The model under review builds one solid part; all positions refer to its coordinate system, in mm. Face numbers are marked on the shaded views. A direction names the side the tool comes from. Coordinates: 2 decimals unless noted, no trailing zeros. Order: outer loops, then holes, each group sorted by start corner. A loop starts at its lowest first (then second) coordinate and runs counter-clockwise, first axis right, second up. Notation, with made-up numbers: M 73,-10.5 L 80,-10.5 A32 ccw 80,23.5 Z; hole C 52.5,76.5 d11. An arc over 180 degrees is marked long. One line per item, written item: value.
```python
from build123d import *

# Parameters (mm, degrees)
SKETCH1_R           = 1.5
BOSS_EXTRUDE1_DEPTH = 2
SKETCH2_R           = 4
SKETCH2_R_2         = 3
BOSS_EXTRUDE2_DEPTH = 3


with BuildPart() as part:
    # Sketch1 → Boss-Extrude1 (new body)
    # profile 1 of 5: a face of its own
    with BuildSketch(Plane(origin=(0, 0, 0), x_dir=(1, 0, 0), z_dir=(0, 1, 0))):
        with BuildLine():
            Line((-3.774917218, 9), (-3.774917218, 4))
            ThreePointArc((-3.774917218, 4), (0, 5.5), (3.774917218, 4))
            Line((3.774917218, 4), (3.774917218, 9))
            Line((3.774917218, 9), (2.5, 17))
            ThreePointArc((2.5, 17), (0, 19.5), (-2.5, 17))
            Line((-2.5, 17), (-3.774917218, 9))
        make_face()
    # profile 2 of 5: a face of its own
    with BuildSketch(Plane(origin=(0, 0, 0), x_dir=(1, 0, 0), z_dir=(0, 1, 0))):
        with BuildLine():
            Line((3.774917218, 4), (-3.774917218, 4))
            ThreePointArc((-3.774917218, 4), (-5.5, 0), (-3.774917218, -4))
            Line((-3.774917218, -4), (3.774917218, -4))
            ThreePointArc((3.774917218, -4), (5.050348735, -2.178067412), (5.5, 0))
            ThreePointArc((5.5, 0), (5.050348735, 2.178067412), (3.774917218, 4))
        make_face()
        with Locations(Location((0, 0, 0), (0, 0, 270))):
            Circle(SKETCH1_R, mode=Mode.SUBTRACT)
    # profile 3 of 5: a face of its own
    with BuildSketch(Plane(origin=(0, 0, 0), x_dir=(1, 0, 0), z_dir=(0, 1, 0))):
        with BuildLine():
            ThreePointArc((3.774917218, 4), (0, 5.5), (-3.774917218, 4))
            Line((-3.774917218, 4), (3.774917218, 4))
        make_face()
    # profile 4 of 5: a face of its own
    with BuildSketch(Plane(origin=(0, 0, 0), x_dir=(1, 0, 0), z_dir=(0, 1, 0))):
        with BuildLine():
            Line((3.774917218, -4), (-3.774917218, -4))
            ThreePointArc((-3.774917218, -4), (0, -5.5), (3.774917218, -4))
        make_face()
    # profile 5 of 5: a face of its own
    with BuildSketch(Plane(origin=(0, 0, 0), x_dir=(1, 0, 0), z_dir=(0, 1, 0))):
        with BuildLine():
            ThreePointArc((3.774917218, -4), (0, -5.5), (-3.774917218, -4))
            Line((-3.774917218, -4), (-3.774917218, -9))
            Line((-3.774917218, -9), (-2.5, -17))
            ThreePointArc((-2.5, -17), (0, -19.5), (2.5, -17))
            Line((2.5, -17), (3.774917218, -9))
            Line((3.774917218, -9), (3.774917218, -4))
        make_face()
    extrude(amount=BOSS_EXTRUDE1_DEPTH)

    # Sketch2 → Boss-Extrude2 (add)
    with BuildSketch(Plane(origin=(0, 2, 0), x_dir=(1, 0, 0), z_dir=(0, 1, 0))):
        with Locations(Location((0, 0, 0), (0, 0, 270))):
            Circle(SKETCH2_R)
        with Locations(Location((0, 0, 0), (0, 0, 270))):
            Circle(SKETCH2_R_2, mode=Mode.SUBTRACT)
    extrude(amount=BOSS_EXTRUDE2_DEPTH)


solid = part.part
```
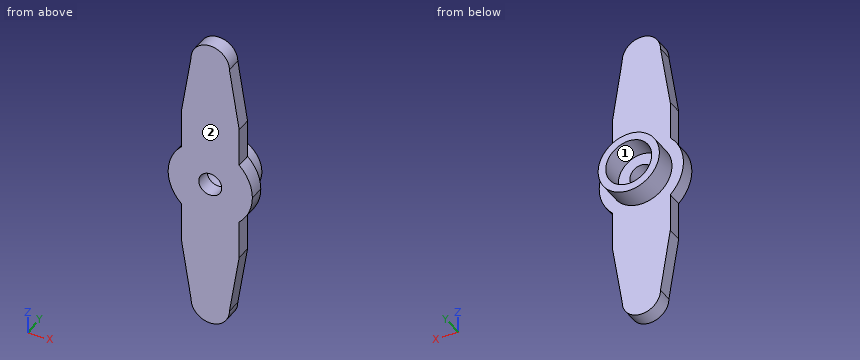
(1) For L1, parallel to X at y = 4, z = 0; L2, parallel to Y at x = -0.5, z = 11; L3, parallel to Z at x = -1, y = 3.55, list the stretches that pass through material, from the lowest coordinate up.
Geometry results:
L1: x = -4 to -3, 3 to 4
L2: y = 0 to 2
L3: z = -3.87 to -2.83, 2.83 to 3.87
(2) Insertion check: pin 1 Ø1.6 at (y, z) = (0.5, -7) entering from -X; pin 2 Ø0.6 at (y, z) = (1, 6) entering from +X; pin 3 Ø1.5 at (x, y) = (2.5, 1.5) entering from +Z; pin 4 Ø2 at (y, z) = (4, 13.5) entering from +X. Each pin has a flat end and moves straight along its axis. Give the tip position at first contact, or say it passes through.
Geometry results:
pin 1: stops at x = -3.77
pin 2: stops at x = 3.77
pin 3: stops at z = 18.79
pin 4: passes through
(3) We need section B-B, the plane z = -0.5. State the section outline as (x, y) points.
Geometry results:
outline: M -5.48,0 L -1.41,0 L -1.41,2 L -2.96,2 L -2.96,5 L -3.97,5 L -3.97,2 L -5.48,2 Z; M 1.41,0 L 5.48,0 L 5.48,2 L 3.97,2 L 3.97,5 L 2.96,5 L 2.96,2 L 1.41,2 Z
(4) We need section D-D, the plane z = -4.5. State the section outline as (x, y) points, plus the area to 3 significant figures.
Geometry results:
outline: M -3.77,0 L 3.77,0 L 3.77,2 L -3.77,2 Z
area: 15.1 mm2
(5) We need section C-C, the plane y = 3.95. State the section outline as (x, z) points, plus the area to 3 significant figures.
Geometry results:
outline: C 0,0 d8; hole C 0,0 d6
area: 22.0 mm2
(6) Tool access review of the marked faces 1 and 2: name each direction out of +Z, -Z, +X, -X, +Y, -Y from which nothing blocks a thin tool from reaching the whole face with its end or side.
Geometry results:
face 1: +Y
face 2: +Z, -Z, +X, -X, -Y
(7) We need section A-A, the plane x = 0. State the section outline as (y, z) points.
Geometry results:
outline: M 0,-19.5 L 2,-19.5 L 2,-4 L 5,-4 L 5,-3 L 2,-3 L 2,-1.5 L 0,-1.5 Z; M 0,1.5 L 2,1.5 L 2,3 L 5,3 L 5,4 L 2,4 L 2,19.5 L 0,19.5 Z
